Part model, mm, in its own coordinate system. Face numbers are marked on the shaded views. A direction names the side the tool comes from. Round coordinates to 2 decimals unless told otherwise and drop trailing zeros. Loops run counter-clockwise (first coordinate to the right, second up) from the corner with the lowest first, then second, coordinate; pieces in that order, holes last.
1) 3-axis set-ups, long thin cutter, end or side, ignore diameter. For the marked faces 4, 5 and 6: which of +Z, -Z, +X, -X, +Y, -Y reach the whole face in a straight line?
2) Band-saw the part on C-C, the plane z = 7.5. Write the cut outline in (x, y).
3) Mould opens along Y. For the marked faces 1, 2 and 3 say: +Y half, -Y half, draft (parallel to the pull), parting line (faces both ways), or undercut.
4) Band-saw the part on D-D, the plane x = 2.5. Write the cut outline in (y, z), then the cut area to 3 significant figures.
5) Band-saw the part on B-B, the plane z = 87. Write the cut outline in (x, y), then the cut area to 3 significant figures.
6) Drop flat-ended pins along their axis: P1, Ø2, axis at y = -12, z = 32.5, coming from the -X side; P2, Ø2, axis at y = -26.5, z = 12, coming from the +X side; P3, Ø5, axis at x = -48, z = 46, coming from the +Y side. Give the stop position or say it passes through.
7) Band-saw the part on A-A, the plane y = -29.75. Write the cut outline in (x, z), then the cut area to 3 significant figures.
8) Probe line 1 (Z direction, x = 7.5, y = -22.25); line 2 (Y direction, x = 34, z = 28); line 3 (Z direction, x = 31, y = -7.75). List the from-to ranges inside material, lowest first.
from build123d import *

# Parameters (mm, degrees)
BOSS_EXTRUDE1_DEPTH = 116
FILLET1_R           = 3
CHAMFER2_SIZE       = 3
CHAMFER2_SIZE_2     = 11.196152423
FILLET2_R           = 0.5
SKETCH3_W           = 3.5
SKETCH3_H           = 7.8
CUT_EXTRUDE1_DEPTH  = 9
SKETCH4_R           = 2.3
CUT_EXTRUDE2_DEPTH  = 161.962973694
CUT_EXTRUDE3_START  = -20
CUT_EXTRUDE3_DEPTH  = 22
CUT_EXTRUDE4_START  = -74
CUT_EXTRUDE4_DEPTH  = 22


with BuildPart() as part:
    # Sketch2 → Boss-Extrude1 (new body)
    with BuildSketch(Plane.XY):
        with BuildLine():
            Line((-39.5, -5.286657915), (-10.5, -5.286657915))
            Line((-10.5, -5.286657915), (-14.035367394, -15))
            Line((-14.035367394, -15), (14.035367394, -15))
            Line((14.035367394, -15), (10.5, -5.286657915))
            Line((10.5, -5.286657915), (39.5, -5.286657915))
            Line((39.5, -5.286657915), (36.005885751, -14.886657915))
            Line((36.005885751, -14.886657915), (53, -14.886657915))
            Line((53, -14.886657915), (53, -34.886657915))
            Line((53, -34.886657915), (16, -34.886657915))
            ThreePointArc((16, -34.886657915), (0, -26.886657915), (-16, -34.886657915))
            Line((-16, -34.886657915), (-53, -34.886657915))
            Line((-53, -34.886657915), (-53, -14.886657915))
            Line((-53, -14.886657915), (-36.005885751, -14.886657915))
            Line((-36.005885751, -14.886657915), (-39.5, -5.286657915))
        make_face()
    extrude(amount=BOSS_EXTRUDE1_DEPTH)

    # Fillet1
    fillet1_edges = [part.edges().sort_by_distance(p)[0] for p in [
        (-53, -24.886657915, 0),
        (53, -24.886657915, 0),
        (-53, -24.886657915, 116),
        (53, -24.886657915, 116),
    ]]
    fillet(fillet1_edges, radius=FILLET1_R)

    # Chamfer2
    # the kernel refuses this chamfer: 11.196152423, 3 mm, written as the material it takes off along each edge
    with BuildSketch(Plane(origin=(50, -34.886657915, 3), x_dir=(1, 0, 0), z_dir=(0, 0, 1))) as chamfer2_piece_1:
        Polygon((3 - CHAMFER2_SIZE, 0), (3, CHAMFER2_SIZE_2), (3, 0), align=None)
    revolve(axis=Axis((50, -34.886657915, 3), (0, 1, 0)), revolution_arc=90, mode=Mode.SUBTRACT)
    with BuildSketch(Plane(origin=(50, -34.886657915, 116), x_dir=(0, 1, 0), z_dir=(-1, 0, 0))) as chamfer2_piece_2:
        Polygon((CHAMFER2_SIZE_2, 0), (0, CHAMFER2_SIZE), (0, 0), align=None)
    extrude(amount=63.073290499, mode=Mode.SUBTRACT)
    with BuildSketch(Plane(origin=(13.073290499, -34.886657915, 0), x_dir=(0, 0, 1), z_dir=(-1, 0, 0))) as chamfer2_piece_3:
        Polygon((CHAMFER2_SIZE, 0), (0, CHAMFER2_SIZE_2), (0, 0), align=None)
    extrude(amount=63.073290499, mode=Mode.SUBTRACT)
    with BuildSketch(Plane(origin=(-50, -34.886657915, 113), x_dir=(-1, 0, 0), z_dir=(0, 0, -1))) as chamfer2_piece_4:
        Polygon((3 - CHAMFER2_SIZE, 0), (3, CHAMFER2_SIZE_2), (3, 0), align=None)
    revolve(axis=Axis((-50, -34.886657915, 113), (0, 1, 0)), revolution_arc=90, mode=Mode.SUBTRACT)
    with BuildSketch(Plane(origin=(-53, -34.886657915, 3), x_dir=(1, 0, 0), z_dir=(0, 0, 1))) as chamfer2_piece_5:
        Polygon((CHAMFER2_SIZE, 0), (0, CHAMFER2_SIZE_2), (0, 0), align=None)
    extrude(amount=110, mode=Mode.SUBTRACT)
    with BuildSketch(Plane(origin=(-50, -34.886657915, 3), x_dir=(-1, 0, 0), z_dir=(0, 0, 1))) as chamfer2_piece_6:
        Polygon((3 - CHAMFER2_SIZE, 0), (3, -CHAMFER2_SIZE_2), (3, 0), align=None)
    revolve(axis=Axis((-50, -34.886657915, 3), (0, -1, 0)), revolution_arc=90, mode=Mode.SUBTRACT)
    with BuildSketch(Plane(origin=(13.073290499, -34.886657915, 116), x_dir=(0, 0, -1), z_dir=(-1, 0, 0))) as chamfer2_piece_7:
        Polygon((CHAMFER2_SIZE, 0), (0, -CHAMFER2_SIZE_2), (0, 0), align=None)
    extrude(amount=63.073290499, mode=Mode.SUBTRACT)
    with BuildSketch(Plane(origin=(50, -34.886657915, 113), x_dir=(1, 0, 0), z_dir=(0, 0, -1))) as chamfer2_piece_8:
        Polygon((3 - CHAMFER2_SIZE, 0), (3, -CHAMFER2_SIZE_2), (3, 0), align=None)
    revolve(axis=Axis((50, -34.886657915, 113), (0, -1, 0)), revolution_arc=90, mode=Mode.SUBTRACT)
    with BuildSketch(Plane(origin=(53, -34.886657915, 3), x_dir=(-1, 0, 0), z_dir=(0, 0, 1))) as chamfer2_piece_9:
        Polygon((CHAMFER2_SIZE, 0), (0, -CHAMFER2_SIZE_2), (0, 0), align=None)
    extrude(amount=110, mode=Mode.SUBTRACT)
    with BuildSketch(Plane(origin=(50, -34.886657915, 0), x_dir=(0, 1, 0), z_dir=(-1, 0, 0))) as chamfer2_piece_10:
        Polygon((CHAMFER2_SIZE_2, 0), (0, -CHAMFER2_SIZE), (0, 0), align=None)
    extrude(amount=63.073290499, mode=Mode.SUBTRACT)

    # Fillet2
    fillet2_edges = [part.edges().sort_by_distance(p)[0] for p in [
        (39.5, -5.286657915, 58),
        (10.5, -5.286657915, 58),
        (-10.5, -5.286657915, 58),
        (-39.5, -5.286657915, 58),
    ]]
    fillet(fillet2_edges, radius=FILLET2_R)

    # Sketch3 → Cut-Extrude1 (cut)
    with BuildSketch(Plane(origin=(0, -5.286657915, 0), x_dir=(1, 0, 0), z_dir=(0, 1, 0))):
        with Locations((-29.285925997, -28)):
            Rectangle(SKETCH3_W, SKETCH3_H)
        with Locations((29.285925997, -28)):
            Rectangle(SKETCH3_W, SKETCH3_H)
    extrude(amount=-CUT_EXTRUDE1_DEPTH, mode=Mode.SUBTRACT)

    # Sketch4 → Cut-Extrude2 (cut, through all)
    with BuildSketch(Plane.ZY.offset(53)):
        with Locations(Location((28, -10.286657915, 0), (0, 0, 270))):
            Circle(SKETCH4_R)
    extrude(amount=-CUT_EXTRUDE2_DEPTH, mode=Mode.SUBTRACT)

    # Sketch5 → Cut-Extrude3 (cut)
    with BuildSketch(Plane(origin=(0, 0, 0), x_dir=(-1, 0, 0), z_dir=(0, 0, -1)).offset(CUT_EXTRUDE3_START)):
        with BuildLine():
            ThreePointArc((9.324082409, -23.690505492), (20.713547019, -32.888480537), (25, -46.886657915))
            ThreePointArc((25, -46.886657915), (-13.998177377, -67.600204934), (-9.324082409, -23.690505492))
            Line((-9.324082409, -23.690505492), (-19.024681673, -23.690505492))
            ThreePointArc((-19.024681673, -23.690505492), (-12.830813493, -74.004368458), (30, -46.886657915))
            ThreePointArc((30, -46.886657915), (27.117710543, -34.055844421), (19.024681673, -23.690505492))
            Line((19.024681673, -23.690505492), (9.324082409, -23.690505492))
        make_face()
        with BuildLine():
            ThreePointArc((-9.324082409, -23.690505492), (0, -21.886657915), (9.324082409, -23.690505492))
            Line((9.324082409, -23.690505492), (19.024681673, -23.690505492))
            ThreePointArc((19.024681673, -23.690505492), (0, -16.886657915), (-19.024681673, -23.690505492))
            Line((-19.024681673, -23.690505492), (-9.324082409, -23.690505492))
        make_face()
    extrude(amount=-CUT_EXTRUDE3_DEPTH, mode=Mode.SUBTRACT)

    # Sketch5<3> → Cut-Extrude4 (cut)
    with BuildSketch(Plane(origin=(0, 0, 0), x_dir=(-1, 0, 0), z_dir=(0, 0, -1)).offset(CUT_EXTRUDE4_START)):
        with BuildLine():
            ThreePointArc((9.324082409, -23.690505492), (20.713547019, -32.888480537), (25, -46.886657915))
            ThreePointArc((25, -46.886657915), (-13.998177377, -67.600204934), (-9.324082409, -23.690505492))
            Line((-9.324082409, -23.690505492), (-19.024681673, -23.690505492))
            ThreePointArc((-19.024681673, -23.690505492), (-12.830813493, -74.004368458), (30, -46.886657915))
            ThreePointArc((30, -46.886657915), (27.117710543, -34.055844421), (19.024681673, -23.690505492))
            Line((19.024681673, -23.690505492), (9.324082409, -23.690505492))
        make_face()
        with BuildLine():
            ThreePointArc((-9.324082409, -23.690505492), (0, -21.886657915), (9.324082409, -23.690505492))
            Line((9.324082409, -23.690505492), (19.024681673, -23.690505492))
            ThreePointArc((19.024681673, -23.690505492), (0, -16.886657915), (-19.024681673, -23.690505492))
            Line((-19.024681673, -23.690505492), (-9.324082409, -23.690505492))
        make_face()
    extrude(amount=-CUT_EXTRUDE4_DEPTH, mode=Mode.SUBTRACT)


solid = part.part
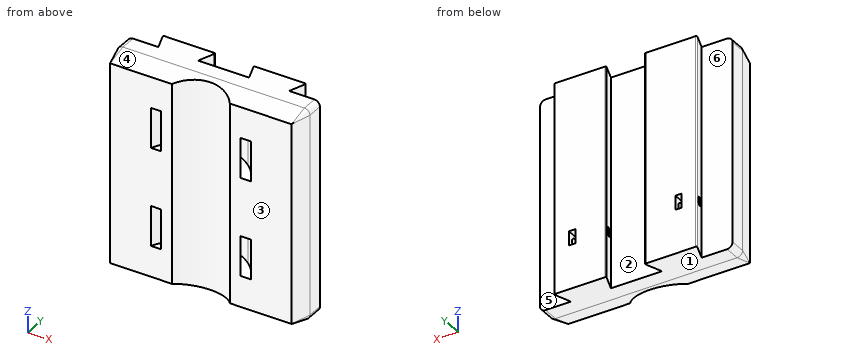
Reported:
1. face 4: +Z, +X, -X, -Y
1. face 5: +Z, -Z, +X
1. face 6: +Z, -Z, -X
2. outline: (-53, -23.69) - (-50, -34.89) - (-16, -34.89) arc R20 cw to (16, -34.89) - (50, -34.89) - (53, -23.69) - (53, -14.89) - (36.01, -14.89) - (39.26, -5.96) arc R0.5 ccw to (38.79, -5.29) - (11.21, -5.29) arc R0.5 ccw to (10.74, -5.96) - (14.04, -15) - (-14.04, -15) - (-10.74, -5.96) arc R0.5 ccw to (-11.21, -5.29) - (-38.79, -5.29) arc R0.5 ccw to (-39.26, -5.96) - (-36.01, -14.89) - (-53, -14.89) - close
3. face 1: draft
3. face 2: undercut
3. face 3: -Y half
4. outline: (-27.04, 0.9) - (-23.69, 0) - (-15, 0) - (-15, 116) - (-23.69, 116) - (-27.04, 115.1) - close; hole (-22.01, 20) - (-16.99, 20) - (-16.99, 42) - (-22.01, 42) - close; hole (-22.01, 74) - (-16.99, 74) - (-16.99, 96) - (-22.01, 96) - close
4. area: 1,170 mm2
5. outline: (-53, -23.69) - (-50, -34.89) - (-27.5, -34.89) arc R30 cw to (27.5, -34.89) - (50, -34.89) - (53, -23.69) - (53, -14.89) - (36.01, -14.89) - (39.26, -5.96) arc R0.5 ccw to (38.79, -5.29) - (11.21, -5.29) arc R0.5 ccw to (10.74, -5.96) - (14.04, -15) - (-14.04, -15) - (-10.74, -5.96) arc R0.5 ccw to (-11.21, -5.29) - (-38.79, -5.29) arc R0.5 ccw to (-39.26, -5.96) - (-36.01, -14.89) - (-53, -14.89) - close; (-21.93, -34.89) - (-16, -34.89) arc R20 cw to (16, -34.89) - (21.93, -34.89) arc R25 ccw to start
5. area: 2,090 mm2
6. P1: stops at x = -37.42
6. P2: stops at x = 52.52
6. P3: stops at y = -14.89
7. outline: (-51.38, 3) arc R1.38 ccw to (-50, 1.62) - (-10.31, 1.62) - (-10.31, 114.38) - (-50, 114.38) arc R1.38 ccw to (-51.38, 113) - close; (10.31, 1.62) - (50, 1.62) arc R1.38 ccw to (51.38, 3) - (51.38, 113) arc R1.38 ccw to (50, 114.38) - (10.31, 114.38) - close; hole (-24.62, 20) - (-18.2, 20) - (-18.2, 42) - (-24.62, 42) - close; hole (-24.62, 74) - (-18.2, 74) - (-18.2, 96) - (-24.62, 96) - close; hole (18.2, 20) - (24.62, 20) - (24.62, 42) - (18.2, 42) - close; hole (18.2, 74) - (24.62, 74) - (24.62, 96) - (18.2, 96) - close
7. area: 8,690 mm2
8. line 1: z = 0 to 20, 42 to 74, 96 to 116
8. line 2: y = -34.89 to -12.59, -7.99 to -5.29
8. line 3: z = 0 to 24.1, 31.9 to 116
